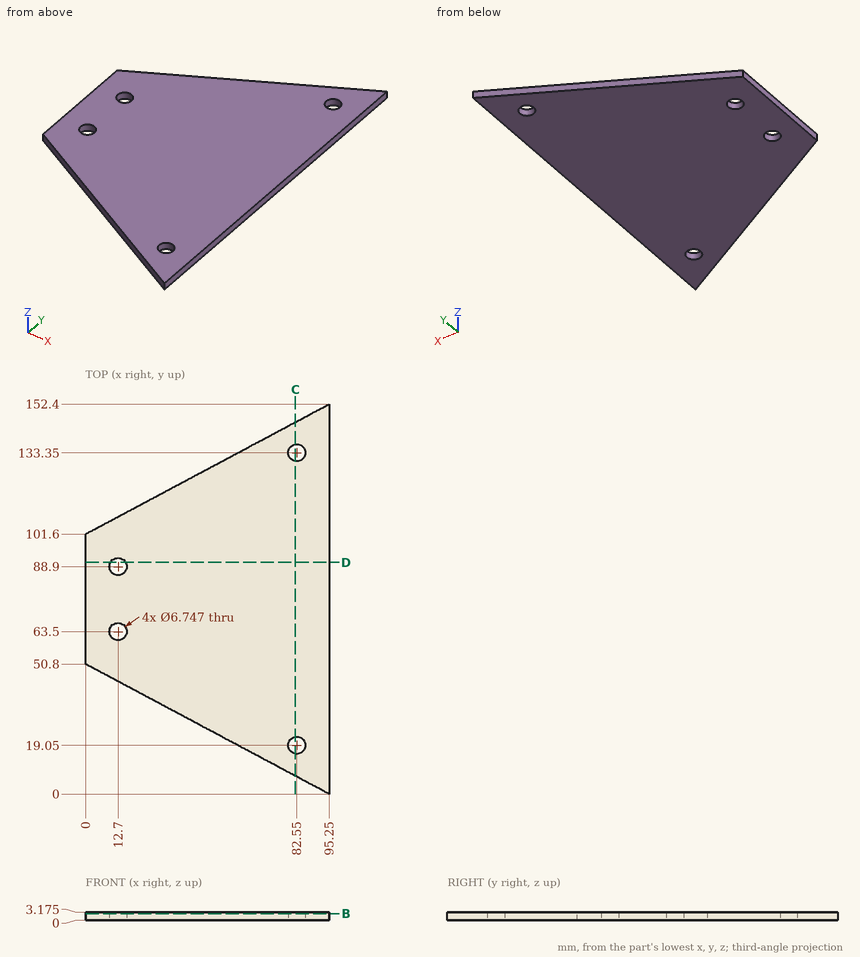
The figure shows three views and two pictorial views of one solid part (mm, origin at its lowest corner). Answer the questions. Round coordinates to 2 decimals unless told otherwise and drop trailing zeros. Write each loop counter-clockwise with the first axis right and the second up, starting at its lowest first coordinate (ties: lowest second). Pieces come first, ordered by that corner, then holes. Notation, with made-up numbers: (-21.5, 8.5) - (18.5, 8.5) arc R21 cw to (18.5, 32.5) - close; hole circle Ø8 at (-27, -10.5). An arc over 180 degrees is marked (long way). One line per question, with ' | ' between items. Start each with the question number.
1. Find the intervals of material crossed by probe 1 along Y at (x, z) = (82.55, 1); probe 2 along Y at (x, z) = (12.7, 1.9); probe 3 along X at (y, z) = (132, 0.4), in increasing order. Write a range as [from, to].
2. Section D-D (y = 90.5) is taken. Determine the outline of the cut face in (x, z) (3 decimals), and give its area (3 significant figures).
3. Section C-C (x = 82) is taken. Determine the outline of the cut face in (y, z) (3 decimals), and give its area (3 significant figures).
4. Section B-B (z = 2.6) is taken. Determine the outline of the cut face in (x, y).
Filled in:
1) probe 1: [6.77, 15.68], [22.42, 129.98], [136.72, 145.63] | probe 2: [44.03, 60.13], [66.87, 85.53], [92.27, 108.37] | probe 3: [57, 79.46], [85.64, 95.25]
2) outline: (0, 0) - (9.73, 0) - (9.73, 3.175) - (0, 3.175) - close; (15.67, 0) - (95.25, 0) - (95.25, 3.175) - (15.67, 3.175) - close | area: 284 mm²
3) outline: (7.067, 0) - (15.722, 0) - (15.722, 3.175) - (7.067, 3.175) - close; (22.378, 0) - (130.022, 0) - (130.022, 3.175) - (22.378, 3.175) - close; (136.678, 0) - (145.333, 0) - (145.333, 3.175) - (136.678, 3.175) - close | area: 397 mm²
4) outline: (0, 50.8) - (95.25, 0) - (95.25, 152.4) - (0, 101.6) - close; hole circle Ø6.75 at (12.7, 63.5); hole circle Ø6.75 at (12.7, 88.9); hole circle Ø6.75 at (82.55, 19.05); hole circle Ø6.75 at (82.55, 133.35)
